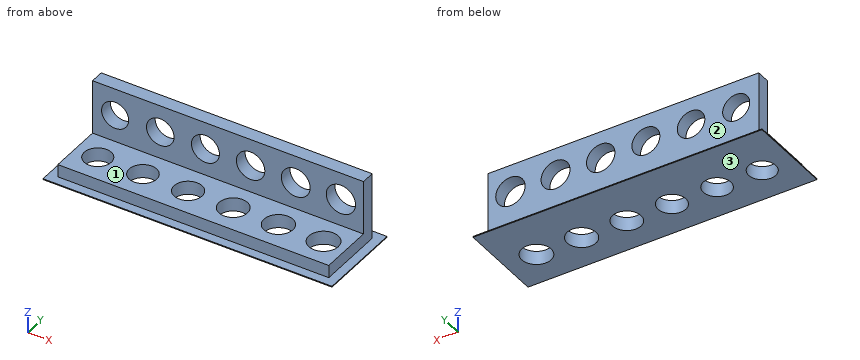
from build123d import *

# Parameters (mm, degrees)
F0_W     = 60
F0_H     = 15
F0_R     = 3
F0_R_2   = 3.05
F0_R_3   = 3.1
F0_R_4   = 3.15
F0_R_5   = 3.2
F0_R_6   = 3.25
F1_DEPTH = 3
F2_W     = 64
F2_H     = 19
F2_W_2   = 60
F2_H_2   = 15
F3_DEPTH = 0.2
F4_W     = 60
F4_H     = 3
F5_DEPTH = 12
F6_R     = 3
F6_R_2   = 3.05
F6_R_3   = 3.1
F6_R_4   = 3.15
F6_R_5   = 3.2
F6_R_6   = 3.25
F7_DEPTH = 3


with BuildPart() as f1:
    # F0 (on Top) → F1 (new body)
    with BuildSketch(Plane.XY):
        with Locations((30, 7.5)):
            Rectangle(F0_W, F0_H)
        with Locations((5, 6)):
            Circle(F0_R, mode=Mode.SUBTRACT)
        with Locations((15, 6)):
            Circle(F0_R_2, mode=Mode.SUBTRACT)
        with Locations((25, 6)):
            Circle(F0_R_3, mode=Mode.SUBTRACT)
        with Locations((35, 6)):
            Circle(F0_R_4, mode=Mode.SUBTRACT)
        with Locations((45, 6)):
            Circle(F0_R_5, mode=Mode.SUBTRACT)
        with Locations((55, 6)):
            Circle(F0_R_6, mode=Mode.SUBTRACT)
    extrude(amount=F1_DEPTH)

    # F2 (on Top) → F3 (join)
    with BuildSketch(Plane.XY):
        with Locations((30, 7.5)):
            Rectangle(F2_W, F2_H)
        with Locations((30, 7.5)):
            Rectangle(F2_W_2, F2_H_2, mode=Mode.SUBTRACT)
    extrude(amount=F3_DEPTH)

    # F4 (on face) → F5 (join)
    with BuildSketch(Plane.XY.offset(3)):
        with Locations((30, 13.5)):
            Rectangle(F4_W, F4_H)
    extrude(amount=F5_DEPTH)

    # F6 (on face) → F7 (cut, through all)
    with BuildSketch(Plane.XZ.offset(-12)):
        with Locations((5, 9)):
            Circle(F6_R)
        with Locations((15, 9)):
            Circle(F6_R_2)
        with Locations((25, 9)):
            Circle(F6_R_3)
        with Locations((35, 9)):
            Circle(F6_R_4)
        with Locations((45, 9)):
            Circle(F6_R_5)
        with Locations((55, 9)):
            Circle(F6_R_6)
    extrude(amount=-F7_DEPTH, mode=Mode.SUBTRACT)


solid = f1.part
The listing builds one solid part. Answer for the finished solid, in the listing's coordinates (mm). Face numbers are marked on the shaded views. A direction names the side the tool comes from. Round coordinates to 2 decimals unless told otherwise and drop trailing zeros. Order: outer loops, then holes, each group sorted by start corner. A loop starts at its lowest first (then second) coordinate and runs counter-clockwise, first axis right, second up. Notation, with made-up numbers: M -30,48 L 0,48 A10 cw 0,53 Z; hole C -13,-26 d2. An arc over 180 degrees is marked long. Answer in a Markdown table with one row per item. Add a question column.
1) The part is cut by section A-A on z = 9. Determine the outline of the cut face in (x, y), plus the area to 3 significant figures.
2) Flat-ended cylindrical pins translate along their axes: pin 1 Ø2 at (x, y) = (26.5, 6) entering from -Z; pin 2 Ø3.5 at (x, y) = (21.5, 5) entering from +Z; pin 3 Ø5 at (x, y) = (12, 10.5) entering from -Z; pin 4 Ø6 at (x, z) = (30, 9.5) entering from -Y. Find the tip coordinate at first contact, or state that the pin passes through.
3) The part is cut by section C-C on y = 6. Count the separate pieces of the cut face and the enclosed holes in it, plus the area to 3 significant figures.
4) The part is cut by section B-B on x = 15. Determine the outline of the cut face in (y, z).
5) Consider line 1 along Y through (x, z) = (15, 1); line 2 along Z through (x, y) = (15, 12.6); line 3 along Z through (x, y) = (55, 13.4). Determine where each line is inside the solid, lowest interval first. Write a range as from..to.
6) The part is cut by section D-D on x = 25. Determine the outline of the cut face in (y, z).
7) Which of the six approach directions +Z, -Z, +X, -X, +Y, -Y give full straight-line access (tool end or side, diameter ignored) to the marked faces 1, 2 and 3?
Findings below:
| question | item | result |
|---|---|---|
| 1 | outline | M 0,12 L 2,12 L 2,15 L 0,15 Z; M 8,12 L 11.95,12 L 11.95,15 L 8,15 Z; M 18.05,12 L 21.9,12 L 21.9,15 L 18.05,15 Z; M 28.1,12 L 31.85,12 L 31.85,15 L 28.1,15 Z; M 38.15,12 L 41.8,12 L 41.8,15 L 38.15,15 Z; M 48.2,12 L 51.75,12 L 51.75,15 L 48.2,15 Z; M 58.25,12 L 60,12 L 60,15 L 58.25,15 Z |
| 1 | area | 67.5 mm² |
| 2 | pin 1 | passes through |
| 2 | pin 2 | stops at z = 3 |
| 2 | pin 3 | stops at z = 0 |
| 2 | pin 4 | stops at y = 12 |
| 3 | separate pieces | 7 |
| 3 | enclosed holes | 0 |
| 3 | area | 68.3 mm² |
| 4 | outline | M -2,0 L 2.95,0 L 2.95,3 L 0,3 L 0,0.2 L -2,0.2 Z; M 9.05,0 L 17,0 L 17,0.2 L 15,0.2 L 15,5.95 L 12,5.95 L 12,3 L 9.05,3 Z; M 12,12.05 L 15,12.05 L 15,15 L 12,15 Z |
| 5 | line 1 | y = 0..2.95, 9.05..15 |
| 5 | line 2 | z = 0..5.95, 12.05..15 |
| 5 | line 3 | z = 0..5.75, 12.25..15 |
| 6 | outline | M -2,0 L 2.9,0 L 2.9,3 L 0,3 L 0,0.2 L -2,0.2 Z; M 9.1,0 L 17,0 L 17,0.2 L 15,0.2 L 15,5.9 L 12,5.9 L 12,3 L 9.1,3 Z; M 12,12.1 L 15,12.1 L 15,15 L 12,15 Z |
| 7 | face 1 | +Z, +X, -X, -Y |
| 7 | face 2 | +Z, +X, -X, +Y |
| 7 | face 3 | -Z, +X, -X, +Y, -Y |
